Read the model definition and answer for the solid it produces. Units are mm, in the model's axes. Face numbers are marked on the shaded views. A direction names the side the tool comes from. Give positions to 0.01 mm unless a question says otherwise; leave off trailing zeros. Order: outer loops, then holes, each group sorted by start corner. A loop starts at its lowest first (then second) coordinate and runs counter-clockwise, first axis right, second up.
```python
from build123d import *

# Parameters (mm, degrees)
MAIN_DEPTH              = 75
ESQUISSE2_R             = 1.5
ENL_V_MAT_EXTRU_1_DEPTH = 8.5
ESQUISSE3_W             = 10
ESQUISSE3_H             = 6.5
ENL_V_MAT_EXTRU_2_DEPTH = 8.5
ESQUISSE4_R             = 1.6
ENL_V_MAT_EXTRU_3_DEPTH = 12


with BuildPart() as part:
    # Esquisse1 → Main (new body)
    with BuildSketch(Plane.XY):
        Polygon((0, 10), (7.5, 10), (7.5, 0), (6.45, 0), (6.45, -1), (3.55, -1), (3.55, 0), (0, 0), align=None)
    extrude(amount=MAIN_DEPTH)

    # Esquisse2 → Enlèv. mat.-Extru.1 (cut, through all)
    with BuildSketch(Plane(origin=(7.5, 0, 0), x_dir=(0, 0, -1), z_dir=(1, 0, 0))):
        with Locations((-5, 7.5)):
            Circle(ESQUISSE2_R)
        with Locations((-70, 7.5)):
            Circle(ESQUISSE2_R)
    extrude(amount=-ENL_V_MAT_EXTRU_1_DEPTH, mode=Mode.SUBTRACT)

    # Esquisse3 → Enlèv. mat.-Extru.2 (cut, through all)
    with BuildSketch(Plane(origin=(7.5, 0, 0), x_dir=(0, 0, -1), z_dir=(1, 0, 0))):
        with Locations((-60, 6.75)):
            Rectangle(ESQUISSE3_W, ESQUISSE3_H)
        with Locations((-15, 6.75)):
            Rectangle(ESQUISSE3_W, ESQUISSE3_H)
    extrude(amount=-ENL_V_MAT_EXTRU_2_DEPTH, mode=Mode.SUBTRACT)

    # Esquisse4 → Enlèv. mat.-Extru.3 (cut, through all)
    with BuildSketch(Plane(origin=(0, -1, 0), x_dir=(-1, 0, 0), z_dir=(0, -1, 0))):
        with Locations((-5, -60)):
            Circle(ESQUISSE4_R)
        with Locations((-5, -15)):
            Circle(ESQUISSE4_R)
    extrude(amount=-ENL_V_MAT_EXTRU_3_DEPTH, mode=Mode.SUBTRACT)


solid = part.part
```
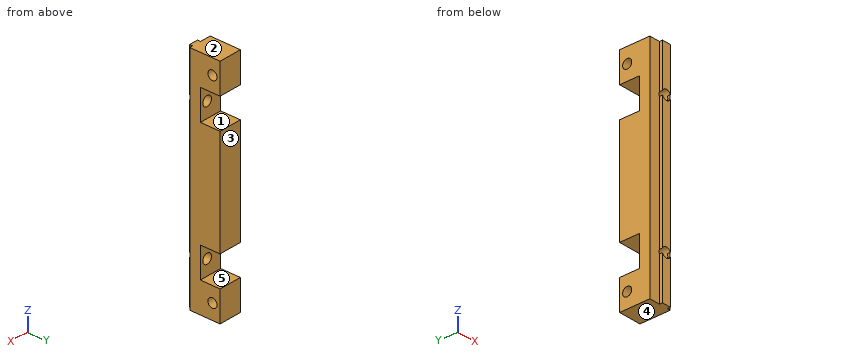
1) Given pin 1 (3 mm diameter, centred on x = 5, z = 15, fed in from -Y); pin 2 (3.5 mm diameter, centred on x = 5, z = 60, fed in from +Y); pin 3 (0.5 mm diameter, centred on y = -0.5, z = 8.5, fed in from -X); pin 4 (0.5 mm diameter, centred on y = -0.5, z = 10.5, fed in from +X), each flat-ended and moving along its own axis, determine where each tip first touches the part or whether it passes through.
Final values:
pin 1: passes through
pin 2: stops at y = 3.5
pin 3: stops at x = 3.55
pin 4: stops at x = 6.45
2) The part is cut by section C-C on x = 1.5. Determine the outline of the cut face in (y, z).
Final values:
outline: (0, 0) - (10, 0) - (10, 10) - (3.5, 10) - (3.5, 20) - (10, 20) - (10, 55) - (3.5, 55) - (3.5, 65) - (10, 65) - (10, 75) - (0, 75) - close; hole circle Ø3 at (7.5, 5); hole circle Ø3 at (7.5, 70)
3) The part is cut by section B-B on y = 7.5. Determine the outline of the cut face in (x, z).
Final values:
outline: (0, 0) - (7.5, 0) - (7.5, 3.5) - (0, 3.5) - close; (0, 6.5) - (7.5, 6.5) - (7.5, 10) - (0, 10) - close; (0, 20) - (7.5, 20) - (7.5, 55) - (0, 55) - close; (0, 65) - (7.5, 65) - (7.5, 68.5) - (0, 68.5) - close; (0, 71.5) - (7.5, 71.5) - (7.5, 75) - (0, 75) - close
4) The part is cut by section D-D on z = 54. Determine the outline of the cut face in (x, y).
Final values:
outline: (0, 0) - (3.55, 0) - (3.55, -1) - (6.45, -1) - (6.45, 0) - (7.5, 0) - (7.5, 10) - (0, 10) - close
5) For a pull along Z with two mould halves and no side action, classify the marked faces 1, 2 and 3 as released by +Z, released by -Z, zero draft, split by the parting line, or undercut.
Final values:
face 1: undercut
face 2: released by +Z
face 3: zero draft
6) Consider L1, parallel to Z at x = 7, y = 9.75; L2, parallel to Z at x = 5, y = 1.65; L3, parallel to X at y = 1.1, z = 60. Determine where each line is inside the solid, lowest interval first.
Final values:
L1: z = 0 to 10, 20 to 55, 65 to 75
L2: z = 0 to 13.4, 16.6 to 58.4, 61.6 to 75
L3: x = 0 to 3.4, 6.6 to 7.5
7) The part is cut by section A-A on z = 5. Determine the outline of the cut face in (x, y), and give its area (3 significant figures).
Final values:
outline: (0, 0) - (3.55, 0) - (3.55, -1) - (6.45, -1) - (6.45, 0) - (7.5, 0) - (7.5, 6) - (0, 6) - close; (0, 9) - (7.5, 9) - (7.5, 10) - (0, 10) - close
area: 55.4 mm2
8) A tool of negligible diameter and unlimited length cuts with its end or side. For the marked faces 4 and 5, from which of +Z, -Z, +X, -X, +Y, -Y can it reach the whole face along a straight path? Write none if from no direction.
Final values:
face 4: -Z, +X, -X, +Y, -Y
face 5: +X, -X, +Y
